Answer from the drawing. Dimensions are ordinates in mm from the lowest x, y and z of the part. A direction names the side the tool comes from. Give positions to 0.01 mm unless a question says otherwise; leave off trailing zeros. Write each loop counter-clockwise with the first axis right and the second up, starting at its lowest first coordinate (ties: lowest second). Pieces come first, ordered by that corner, then holes.
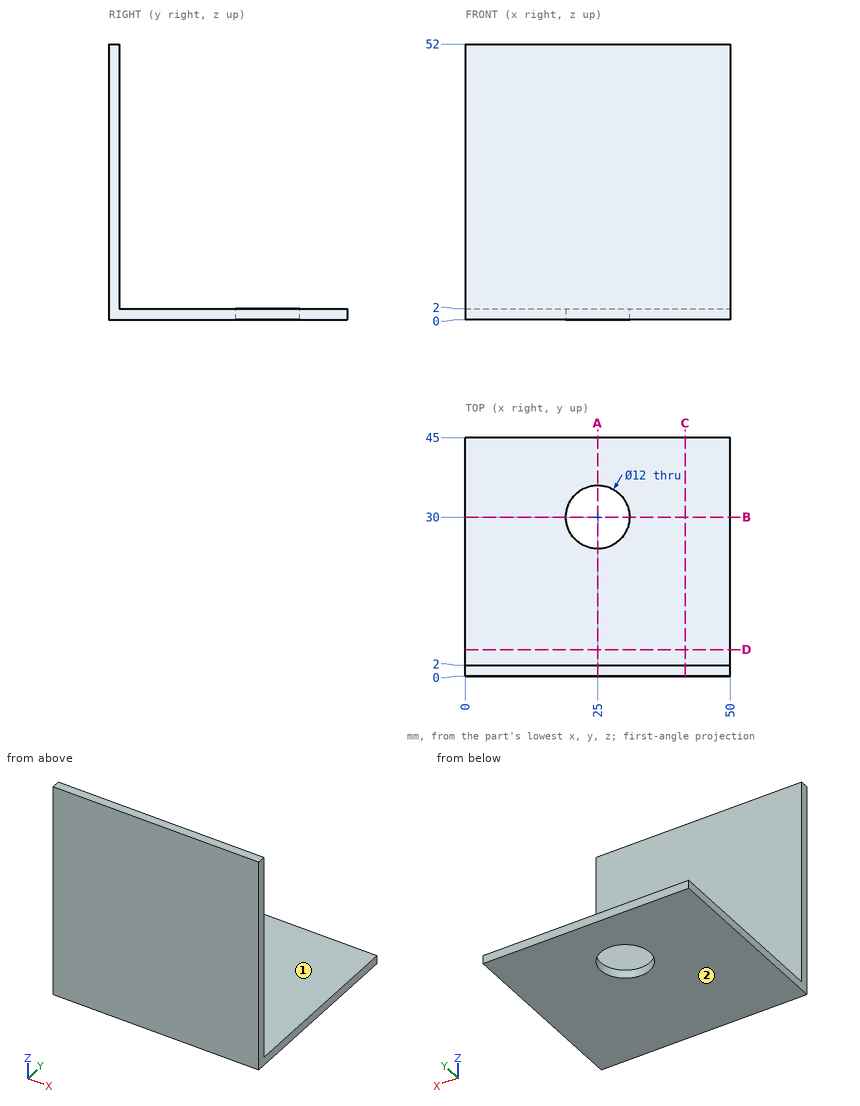
Item 1: A cutting plane is placed at C-C, the plane x = 41.5. Give the vertices of the cut face in (y, z).
Conclusion:
outline: (0, 0) - (45, 0) - (45, 2) - (2, 2) - (2, 52) - (0, 52) - close
Item 2: Which of the six approach directions +Z, -Z, +X, -X, +Y, -Y give full straight-line access (tool end or side, diameter ignored) to the marked faces 1 and 2?
Conclusion:
face 1: +Z, +X, -X, +Y
face 2: -Z, +X, -X, +Y, -Y
Item 3: Consider probe 1 along Y at (x, z) = (25, 1); probe 2 along Z at (x, y) = (9, 17). Determine where each line is inside the solid, lowest interval first.
Conclusion:
probe 1: y = 0 to 24, 36 to 45
probe 2: z = 0 to 2
Item 4: A cutting plane is placed at A-A, the plane x = 25. Give the vertices of the cut face in (y, z).
Conclusion:
outline: (0, 0) - (24, 0) - (24, 2) - (2, 2) - (2, 52) - (0, 52) - close; (36, 0) - (45, 0) - (45, 2) - (36, 2) - close
Item 5: A cutting plane is placed at D-D, the plane y = 5. Give the vertices of the cut face in (x, z).
Conclusion:
outline: (0, 0) - (50, 0) - (50, 2) - (0, 2) - close
Item 6: Each of these flat-tipped pins is pushed along its axis until it touches: P1, Ø2, axis at x = 26.5, z = 10.5, coming from the +Y side; P2, Ø19, axis at x = 25, y = 30, coming from the -Z side; P3, Ø2, axis at x = 8.5, y = 28.5, coming from the +Z side. Where does it stop, or does it pass through?
Conclusion:
P1: stops at y = 2
P2: stops at z = 0
P3: stops at z = 2
Item 7: A cutting plane is placed at B-B, the plane y = 30. Give the vertices of the cut face in (x, z), plus the area to 3 significant figures.
Conclusion:
outline: (0, 0) - (19, 0) - (19, 2) - (0, 2) - close; (31, 0) - (50, 0) - (50, 2) - (31, 2) - close
area: 76.0 mm2
